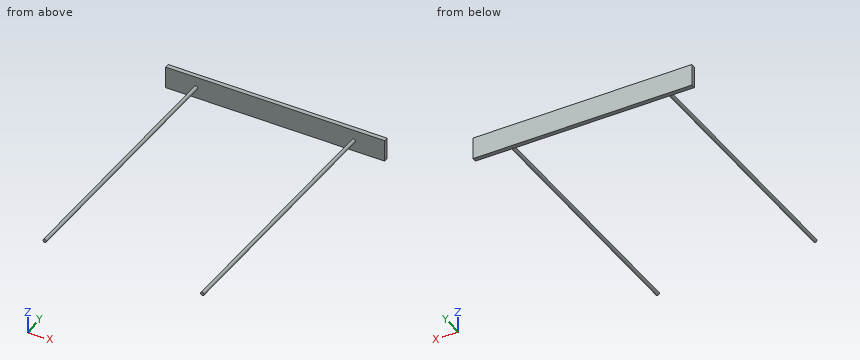
```python
from build123d import *

# Parameters (mm, degrees)
SKETCH1_W           = 500
SKETCH1_H           = 50
BOSS_EXTRUDE1_DEPTH = 10
SKETCH2_R           = 4
BOSS_EXTRUDE2_DEPTH = 600
SKETCH6_R           = 4
BOSS_EXTRUDE3_DEPTH = 600


with BuildPart() as part:
    # Sketch1 → Boss-Extrude1 (new body)
    with BuildSketch(Plane(origin=(0, 0, 0), x_dir=(1, 0, 0), z_dir=(0, 1, 0))):
        Rectangle(SKETCH1_W, SKETCH1_H)
    extrude(amount=BOSS_EXTRUDE1_DEPTH)

    # Sketch2 → Boss-Extrude2 (add)
    with BuildSketch(Plane.XZ):
        with Locations((180, 0)):
            Circle(SKETCH2_R)
    extrude(amount=BOSS_EXTRUDE2_DEPTH)

    # Sketch6 → Boss-Extrude3 (add)
    with BuildSketch(Plane.XZ):
        with Locations((-180, 0)):
            Circle(SKETCH6_R)
    extrude(amount=BOSS_EXTRUDE3_DEPTH)


solid = part.part
```
The listing builds one solid part. Answer for the finished solid, in the listing's coordinates (mm). Give positions to 0.01 mm unless a question says otherwise; leave off trailing zeros. Order: outer loops, then holes, each group sorted by start corner. A loop starts at its lowest first (then second) coordinate and runs counter-clockwise, first axis right, second up. Notation, with made-up numbers: M 72,32.25 L 101,32.25 A5 cw 101,37.25 Z; hole C -8.5,43 d10. An arc over 180 degrees is marked long. Put each result on its own line as item: value. Start each with the question number.
Item 1: Flat-ended cylindrical pins translate along their axes: P1, Ø2, axis at x = 178.5, y = -134.5, coming from the +Z side; P2, Ø5, axis at y = -104, z = 4.5, coming from the +X side; P3, Ø5, axis at x = -72, z = 16, coming from the -Y side. Find the tip coordinate at first contact, or state that the pin passes through.
Item 2: Find the intervals of material crossed by line 1 along Y through (x, z) = (47, -2); line 2 along Z through (x, y) = (182.5, -230); line 3 along Z through (x, y) = (178.5, -80), in increasing order.
Item 3: The part is cut by section C-C, the plane x = -5.5. Determine the outline of the cut face in (y, z).
Item 4: The part is cut by section A-A, the plane y = -144. Determine the outline of the cut face in (x, z).
Item 5: The part is cut by section B-B, the plane z = -16. Determine the outline of the cut face in (x, y).
Answer key:
1. P1: stops at z = 3.97
1. P2: stops at x = 183.46
1. P3: stops at y = 0
2. line 1: y = 0 to 10
2. line 2: z = -3.12 to 3.12
2. line 3: z = -3.71 to 3.71
3. outline: M 0,-25 L 10,-25 L 10,25 L 0,25 Z
4. outline: C -180,0 d8; C 180,0 d8
5. outline: M -250,0 L 250,0 L 250,10 L -250,10 Z
